from build123d import *

# Parameters (mm, degrees)
EXTRUDE_1_DEPTH     = 10
SKETCH_2_W          = 25
SKETCH_2_H          = 25
SKETCH_2_R          = 1.1
CUT_EXTRUDE_1_DEPTH = 8
SKETCH_2_3_R        = 1.1
CUT_EXTRUDE_2_DEPTH = 235.520787991
SKETCH_3_W          = 25
SKETCH_3_H          = 25
CUT_EXTRUDE_3_DEPTH = 235.520787991
FILLET_2_R          = 2


with BuildPart() as part:
    # Sketch 1 → Extrude 1 (new body)
    with BuildSketch(Plane(origin=(0, 0, 0), x_dir=(1, 0, 0), z_dir=(0, 1, 0))):
        Polygon((-150, -120), (20, -120), (20, -180), (80, -180), (80, -120), (150, -120), (150, 120), (-150, 120), align=None)
    extrude(amount=EXTRUDE_1_DEPTH)

    # Sketch 2 → Cut-Extrude 1 (cut)
    with BuildSketch(Plane.XZ):
        with Locations((50, 140)):
            Rectangle(SKETCH_2_W, SKETCH_2_H)
        with Locations(Location((58, 148, 0), (0, 0, 270))):
            Circle(SKETCH_2_R, mode=Mode.SUBTRACT)
        with Locations(Location((42, 148, 0), (0, 0, 270))):
            Circle(SKETCH_2_R, mode=Mode.SUBTRACT)
        with Locations(Location((42, 132, 0), (0, 0, 270))):
            Circle(SKETCH_2_R, mode=Mode.SUBTRACT)
        with Locations(Location((58, 132, 0), (0, 0, 270))):
            Circle(SKETCH_2_R, mode=Mode.SUBTRACT)
    extrude(amount=-CUT_EXTRUDE_1_DEPTH, mode=Mode.SUBTRACT)

    # Sketch 2_3 → Cut-Extrude 2 (cut, through all)
    with BuildSketch(Plane.XZ):
        with Locations(Location((42, 132, 0), (0, 0, 270))):
            Circle(SKETCH_2_3_R)
        with Locations(Location((42, 148, 0), (0, 0, 270))):
            Circle(SKETCH_2_3_R)
        with Locations(Location((58, 132, 0), (0, 0, 270))):
            Circle(SKETCH_2_3_R)
        with Locations(Location((58, 148, 0), (0, 0, 270))):
            Circle(SKETCH_2_3_R)
    extrude(amount=-CUT_EXTRUDE_2_DEPTH, mode=Mode.SUBTRACT)

    # Sketch 3 → Cut-Extrude 3 (cut, through all)
    with BuildSketch(Plane(origin=(0, 10, 0), x_dir=(1, 0, 0), z_dir=(0, 1, 0))):
        with Locations((-17.5, 25)):
            Rectangle(SKETCH_3_W, SKETCH_3_H)
        with Locations((-17.5, -45)):
            Rectangle(SKETCH_3_W, SKETCH_3_H)
        with Locations((-17.5, 60)):
            Rectangle(SKETCH_3_W, SKETCH_3_H)
        with Locations((-17.5, -10)):
            Rectangle(SKETCH_3_W, SKETCH_3_H)
        with Locations((17.5, -45)):
            Rectangle(SKETCH_3_W, SKETCH_3_H)
        with Locations((17.5, -10)):
            Rectangle(SKETCH_3_W, SKETCH_3_H)
        with Locations((17.5, 25)):
            Rectangle(SKETCH_3_W, SKETCH_3_H)
        with Locations((17.5, 60)):
            Rectangle(SKETCH_3_W, SKETCH_3_H)
    extrude(amount=-CUT_EXTRUDE_3_DEPTH, mode=Mode.SUBTRACT)

    # Fillet 2
    fillet_2_edges = [part.edges().sort_by_distance(p)[0] for p in [
        (37.5, 4, 152.5),
        (62.5, 4, 152.5),
        (62.5, 4, 127.5),
        (37.5, 4, 127.5),
    ]]
    fillet(fillet_2_edges, radius=FILLET_2_R)


solid = part.part
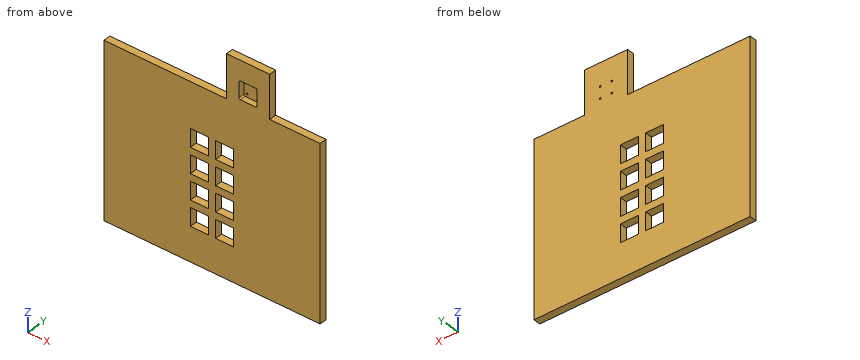
CAD build for the part. Positions are in the model's coordinates, mm. Coordinates: 2 decimals unless noted, no trailing zeros. Write each loop counter-clockwise with the first axis right and the second up, starting at its lowest first coordinate (ties: lowest second). Pieces come first, ordered by that corner, then holes. Notation, with made-up numbers: (38, -25.75) - (66, -25.75) arc R20 cw to (66, -6.75) - close; hole circle Ø2 at (-11, -14.5). An arc over 180 degrees is marked (long way). Use a Markdown table: item, result. Add a question column.
Item 1: Band-saw the part on A-A, the plane x = -36. Give the cut face in (y, z), and give its area (3 significant figures).
Item 2: Drill centre lines: L1, parallel to X at y = 9.2, z = 132; L2, parallel to X at y = 7.25, z = 48.5; L3, parallel to X at y = 4.5, z = 148. Where is each one in solid material? Low to high. Write a range as from..to.
Item 3: Band-saw the part on B-B, the plane y = 2.5. Give the number of separate pieces and of enclosed holes in the cut face, and give its area (3 significant figures).
Item 4: Flat gauge pin, fed straight in: pin 1 (1 mm diameter, centred on x = 106.5, y = 4.5, fed in from +Z). Where does the tip first touch, or does it go through?
Numbers:
| question | item | result |
|---|---|---|
| 1 | outline | (0, -120) - (10, -120) - (10, 120) - (0, 120) - close |
| 1 | area | 2,400 mm2 |
| 2 | L1 | 20..40.9, 43.1..56.9, 59.1..80 |
| 2 | L2 | -150..-30, -5..5, 30..150 |
| 2 | L3 | 20..37.5, 62.5..80 |
| 3 | separate pieces | 1 |
| 3 | enclosed holes | 9 |
| 3 | area | 70,000 mm2 |
| 4 | pin 1 | z = 120 |
